from build123d import *

# Parameters (mm, degrees)
F1_DEPTH    = 30
F2_T1_DEPTH = 30


# Not quite as in the source:
# - a fillet or chamfer that OpenCascade refuses, or shapes differently, is made with other operations: its cross-section is extruded or revolved along the edge and cut away or added
# - ends of sketch curves that miss each other by under 0.0002 mm in the source are joined
# - a feature names something its author has since deleted; it is built from what else it names


with BuildPart() as f1:
    # F0 (on Top) → F1 (new body)
    with BuildSketch(Plane.XY):
        with BuildLine():
            ThreePointArc((0.0090084839, 3.9999898559), (3.7308371777, 1.442516535), (2.6975556514, -2.9535052916))
            Line((2.6975556514, -2.9535052916), (3.4413844377, -3.6272404321))
            ThreePointArc((3.4413844377, -3.6272404321), (4.562894469, -2.0445033784), (4.9976265844, -0.1540406522))
            ThreePointArc((4.9976265844, -0.1540406522), (4.9982482299, -0.0770116198), (5, 0))
            ThreePointArc((5, 0), (4.4620948533, 2.2560384571), (2.964116192, 4.0266630354))
            Line((2.964116192, 4.0266630354), (0.0090084839, 3.9999898559))
        make_face()
        with BuildLine():
            ThreePointArc((-2.6975556514, -2.9535052916), (-3.7275789944, 1.4509151734), (0.0090084839, 3.9999898559))
            Line((0.0090084839, 3.9999898559), (2.964116192, 4.0266630354))
            ThreePointArc((2.964116192, 4.0266630354), (1.5599174374, 4.7504376207), (0, 5))
            ThreePointArc((0, 5), (-2.1802578035, 4.4996084175), (-3.9241225459, 3.0985903642))
            ThreePointArc((-3.9241225459, 3.0985903642), (-4.9871708669, -0.3579479625), (-3.4413844377, -3.6272404321))
            Line((-3.4413844377, -3.6272404321), (-2.6975556514, -2.9535052916))
        make_face()
        with BuildLine():
            ThreePointArc((0, 5), (1.5599174374, 4.7504376207), (2.964116192, 4.0266630354))
            Line((2.964116192, 4.0266630354), (7.1272566982, 4.0641686172))
            ThreePointArc((7.1272566982, 4.0641686172), (8.5825190892, 4.8210552933), (10.200330031, 5.0918944033))
            Line((10.200330031, 5.0918944033), (0, 5))
        make_face()
        with BuildLine():
            ThreePointArc((5, 0), (4.9982482299, -0.0770116198), (4.9976265844, -0.1540406522))
            ThreePointArc((4.9976265844, -0.1540406522), (4.9994066109, -0.0770294678), (5, 0))
        make_face()
        with BuildLine():
            ThreePointArc((5, 0), (4.9994066109, -0.0770294678), (4.9976265844, -0.1540406522))
            ThreePointArc((4.9976265844, -0.1540406522), (5.3752392401, -2.1129770441), (6.4564240892, -3.7895993711))
            Line((6.4564240892, -3.7895993711), (7.1655909773, -3.0842495499))
            ThreePointArc((7.1655909773, -3.0842495499), (6.3350165087, 1.5016234688), (10.2093385862, 4.0919349811))
            Line((10.2093385862, 4.0919349811), (7.1272566982, 4.0641686172))
            ThreePointArc((7.1272566982, 4.0641686172), (5.5962602055, 2.2767129418), (5, 0))
        make_face()
        with BuildLine():
            ThreePointArc((-3.9241225459, 3.0985903642), (-2.1802578035, 4.4996084175), (0, 5))
            Line((0, 5), (-3.9241225459, 5))
            Line((-3.9241225459, 5), (-3.9241225459, 3.0985903642))
        make_face()
        with BuildLine():
            ThreePointArc((10.200330031, 5.0918944033), (8.5825190892, 4.8210552933), (7.1272566982, 4.0641686172))
            Line((7.1272566982, 4.0641686172), (10.2093385862, 4.0919349811))
            Line((10.2093385862, 4.0919349811), (13.2914205601, 4.1197013458))
            ThreePointArc((13.2914205601, 4.1197013458), (11.8227579499, 4.8502464877), (10.200330031, 5.0918944033))
        make_face()
        with BuildLine():
            Line((14.2744146958, 5.1285976842), (10.200330031, 5.0918944033))
            ThreePointArc((10.200330031, 5.0918944033), (11.8227579499, 4.8502464877), (13.2914205601, 4.1197013458))
            ThreePointArc((13.2914205601, 4.1197013458), (13.8120129481, 3.6966683449), (14.2744146958, 3.2107074637))
            Line((14.2744146958, 3.2107074637), (14.2744146958, 5.1285976842))
        make_face()
        with BuildLine():
            Line((13.2914205601, 4.1197013458), (10.2093385862, 4.0919349811))
            ThreePointArc((10.2093385862, 4.0919349811), (14.145125137, 1.5368032872), (13.3296593654, -3.0842495499))
            Line((13.3296593654, -3.0842495499), (14.0388262535, -3.7895993711))
            ThreePointArc((14.0388262535, -3.7895993711), (15.4946546383, -0.3344761776), (14.2744146958, 3.2107074637))
            ThreePointArc((14.2744146958, 3.2107074637), (13.8120129481, 3.6966683449), (13.2914205601, 4.1197013458))
        make_face()
        with BuildLine():
            Line((7.1272566982, 4.0641686172), (2.964116192, 4.0266630354))
            ThreePointArc((2.964116192, 4.0266630354), (4.4620948533, 2.2560384571), (5, 0))
            ThreePointArc((5, 0), (5.5962602055, 2.2767129418), (7.1272566982, 4.0641686172))
        make_face()
    extrude(amount=F1_DEPTH)

    # F2: fillet of radius 1 on 1 edges, made by hand

    # F2_s2 → F2_t1 (join)
    with BuildSketch(Plane.XY):
        with BuildLine():
            ThreePointArc((0.0045042077, 5.0000405782), (-4.57e-08, 5.0000101446), (-0.0045043905, 5))
            Line((-0.0045043905, 5), (0, 5))
            Line((0, 5), (0.0045042077, 5.0000405782))
        make_face()
    extrude(amount=F2_T1_DEPTH)


solid = f1.part
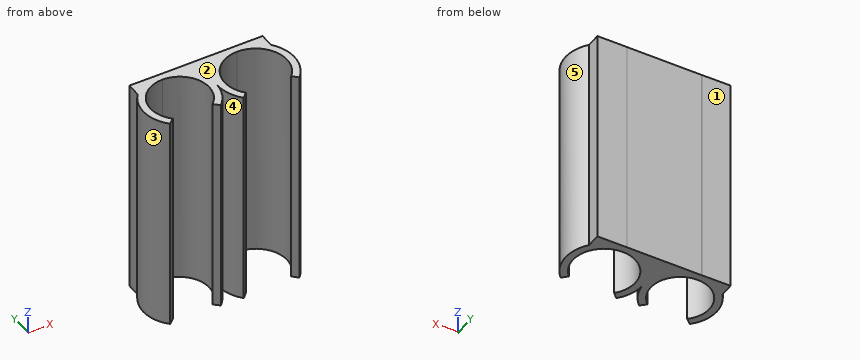
Can you work these out from the model? Positions are in its coordinate system, mm. Face numbers are marked on the shaded views. A direction names the side the tool comes from. Coordinates: 2 decimals unless noted, no trailing zeros. Loops run counter-clockwise (first coordinate to the right, second up) from the corner with the lowest first, then second, coordinate; pieces in that order, holes last. Notation, with made-up numbers: M 60.25,-18.5 L 100.25,-18.5 A13 cw 100.25,5.5 Z; hole C 48.25,23 d9. An arc over 180 degrees is marked long. Answer as CSV lines item,"result". Start each with the question number.
1. For the marked faces 1 and 2, which set-ups out of +Z, -Z, +X, -X, +Y, -Y let a thin tool reach every point of the face, with its end or its side?
2. Suppose I cut it at A-A, the plane y = -2.5. List the corners of the cut face in (x, z) for me.
3. Suppose I cut it at C-C, the plane y = 1.5. List the corners of the cut face in (x, z) for me, plus the area to 3 significant figures.
4. If I drill on probe 1 along X at (y, z) = (0, 10.25); probe 2 along X at (y, z) = (1.25, 17); probe 3 along X at (y, z) = (-1.5, 2.25), over which ranges is the centre line in solid material (lowest first)? Write a range as [from, to].
5. For pin 1 Ø4 at (x, z) = (-2, 9.5) entering from -Y; pin 2 Ø2 at (y, z) = (4, 22) entering from -X; pin 3 Ø1 at (y, z) = (3.5, 21.5) entering from +X; pin 4 Ø1.5 at (x, y) = (1.5, 0.5) entering from +Z, each with a flat end and sliding along its axis, tell me the tip position at first contact or that it passes through.
6. Suppose I cut it at D-D, the plane x = 11.75. List the corners of the cut face in (y, z) for me.
7. Thinking about a two-plate mould opening in X: for the marked faces 3, 4 and 5, which applies, +X half, -X half, draft (parallel to the pull), parting line (faces both ways), or undercut?
Output:
1,face 1,"+Z, -Z, -X, +Y"
1,face 2,"+Z, +X, -X, +Y, -Y"
2,outline,"M -4.33,0 L -3.12,0 L -3.12,30 L -4.33,30 Z; M 3.12,0 L 4.33,0 L 4.33,30 L 3.12,30 Z; M 5.55,0 L 6.7,0 L 6.7,30 L 5.55,30 Z; M 13.79,0 L 14.95,0 L 14.95,30 L 13.79,30 Z"
3,outline,"M -4.77,0 L -3.71,0 L -3.71,30 L -4.77,30 Z; M 3.71,0 L 6.33,0 L 6.33,30 L 3.71,30 Z; M 14.16,0 L 15.23,0 L 15.23,30 L 14.16,30 Z"
3,area,"143 mm^2"
4,probe 1,"x = [-5, -4], [4, 6], [14.49, 15.5]"
4,probe 2,"x = [-4.84, -3.8], [3.8, 6.24], [14.26, 15.31]"
4,probe 3,"x = [-4.77, -3.71], [3.71, 4.77], [5.17, 6.22], [14.28, 15.32]"
5,pin 1,"stops at y = -3.63"
5,pin 2,"stops at x = -4"
5,pin 3,"stops at x = 14.44"
5,pin 4,"passes through"
6,outline,"M 3.82,0 L 5.11,0 L 5.11,30 L 3.82,30 Z"
7,face 3,"-X half"
7,face 4,"undercut"
7,face 5,"+X half"
